Answer from the drawing. Dimensions are ordinates in mm from the lowest x, y and z of the part. Round coordinates to 2 decimals unless told otherwise and drop trailing zeros. Write each loop counter-clockwise with the first axis right and the second up, starting at its lowest first coordinate (ties: lowest second). Pieces come first, ordered by that corner, then holes.
1. Find section A-A (y = 49). Write down the section's boundary in (x, z), and give its area (3 significant figures).
2. Straight lines are drawn through the part: probe 1 along X at (y, z) = (44, 2.3); probe 2 along Y at (x, z) = (45, 4.65). For each, find the intervals that lie inside material, in ascending order.
3. Find section B-B (x = 21). Write down the section's boundary in (y, z), and give its area (3 significant figures).
4. Find section C-C (z = 0.9). Write down the section's boundary in (x, y).
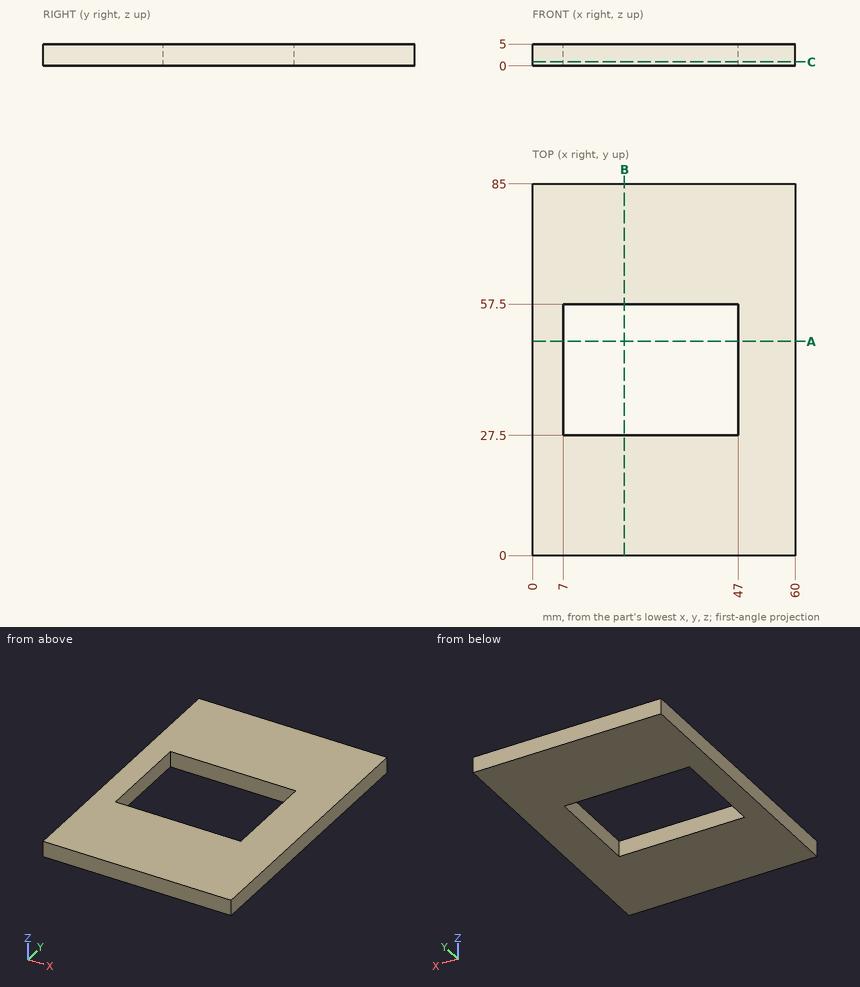
Worked answers:
1. outline: (0, 0) - (7, 0) - (7, 5) - (0, 5) - close; (47, 0) - (60, 0) - (60, 5) - (47, 5) - close
1. area: 100 mm2
2. probe 1: x = 0 to 7, 47 to 60
2. probe 2: y = 0 to 27.5, 57.5 to 85
3. outline: (0, 0) - (27.5, 0) - (27.5, 5) - (0, 5) - close; (57.5, 0) - (85, 0) - (85, 5) - (57.5, 5) - close
3. area: 275 mm2
4. outline: (0, 0) - (60, 0) - (60, 85) - (0, 85) - close; hole (7, 27.5) - (47, 27.5) - (47, 57.5) - (7, 57.5) - close
